Verification items for this drawing (mm, ordinates from the low corner). Coordinates: 2 decimals unless noted, no trailing zeros. Order: outer loops, then holes, each group sorted by start corner. A loop starts at its lowest first (then second) coordinate and runs counter-clockwise, first axis right, second up. Notation, with made-up numbers: (12, -24.5) - (70, -24.5) arc R19 ccw to (70, -15.5) - close; hole circle Ø7 at (41, 13). An arc over 180 degrees is marked (long way). Use CSV: the item, a comma, the result in double quotes. Start each with the question number.
1) Sectioned sample at A-A, the plane z = 10.5. Record the cut outline in (x, y).
2) Draft check along Y on the marked faces 1, 2 and 3. Enter one of: released by +Y, released by -Y, zero draft, split by the parting line, or undercut.
3) Sectioned sample at D-D, the plane z = 3.5. Record the cut outline in (x, y).
4) Sectioned sample at B-B, the plane x = 19. Record the cut outline in (y, z).
5) Depth check by flat-ended pin: P1, Ø6, axis at x = 61.5, y = 43.5, coming from the +Z side; P2, Ø1.8, axis at y = 127.5, z = 3.5, coming from the -X side; P3, Ø3, axis at x = 60, z = 8.5, coming from the +Y side. Enter the tip coordinate at first touch or a pass-through.
6) Thickness scan on probe 1 along Y at (x, z) = (36.5, 13); probe 2 along X at (y, z) = (50.5, 9.75); probe 3 along Y at (x, z) = (37.5, 6.5). Record the ranges inside material, lowest first. Write a range as [from, to].
7) Sectioned sample at C-C, the plane y = 42. Record the cut outline in (x, z).
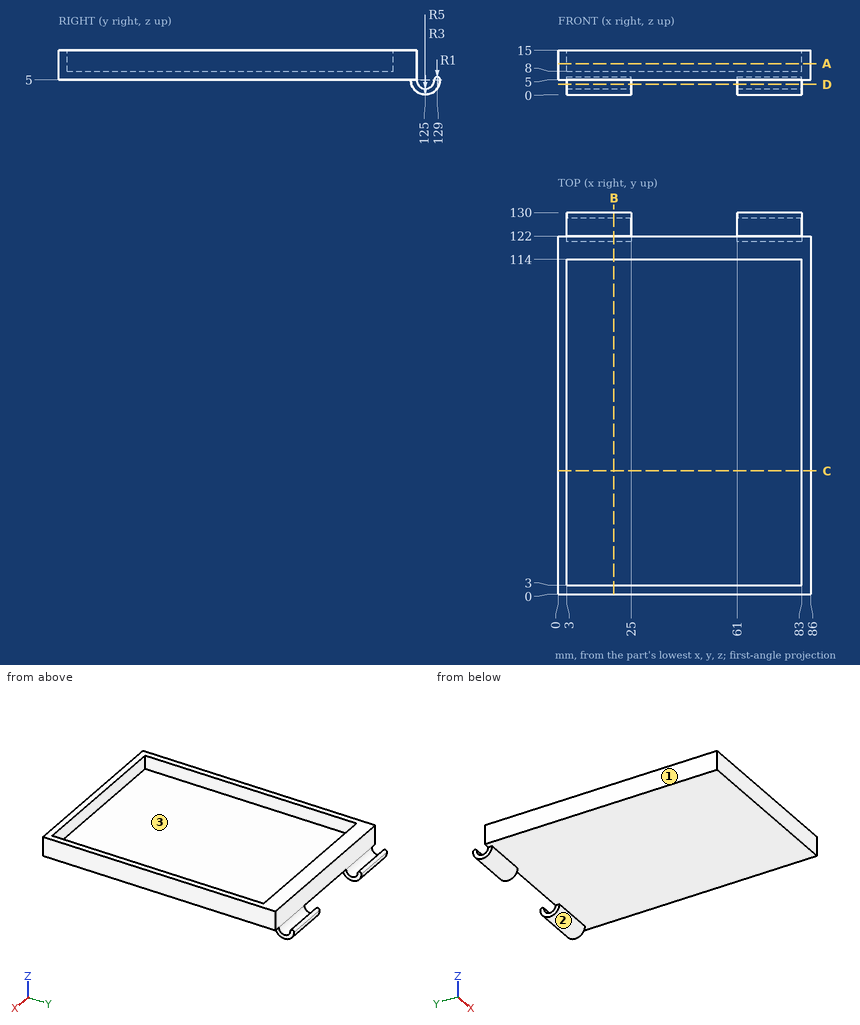
Evaluation:
1,outline,"(0, 0) - (86, 0) - (86, 122) - (0, 122) - close; hole (3, 3) - (83, 3) - (83, 114) - (3, 114) - close"
2,face 1,"zero draft"
2,face 2,"split by the parting line"
2,face 3,"undercut"
3,outline,"(3, 120.23) - (25, 120.23) - (25, 122.4) - (3, 122.4) - close; (3, 127.6) - (25, 127.6) - (25, 129.77) - (3, 129.77) - close; (61, 120.23) - (83, 120.23) - (83, 122.4) - (61, 122.4) - close; (61, 127.6) - (83, 127.6) - (83, 129.77) - (61, 129.77) - close"
4,outline,"(0, 5) - (120, 5) arc R5 ccw to (130, 5) arc R1 ccw to (128, 5) arc R3 cw to (122, 5) - (122, 15) - (114, 15) - (114, 8) - (3, 8) - (3, 15) - (0, 15) - close"
5,P1,"z = 8"
5,P2,"x = 3"
5,P3,"y = 122"
6,probe 1,"[0, 3], [114, 122]"
6,probe 2,"[0, 3], [83, 86]"
6,probe 3,"[0, 122]"
7,outline,"(0, 5) - (86, 5) - (86, 15) - (83, 15) - (83, 8) - (3, 8) - (3, 15) - (0, 15) - close"
